Verification items for the finished model (mm, model axes). Face numbers are marked on the shaded views. A direction names the side the tool comes from. Coordinates: 2 decimals unless noted, no trailing zeros. Write each loop counter-clockwise with the first axis right and the second up, starting at its lowest first coordinate (ties: lowest second). Pieces come first, ordered by that corner, then holes. Notation, with made-up numbers: (7, -19) -> (12, -19) arc R32 ccw to (12, 12) -> close; hole circle Ø10 at (49, 45). An arc over 180 degrees is marked (long way). Write item = value, one per line. Start each with the question number.
(1) Mould release check, pull along Y, two halves, no side actions. Record for the marked faces 3, 4, 5 and 6: released by +Y, released by -Y, zero draft, split by the parting line, or undercut.
(2) Section check B-B (x = 11). Record the cut outline in (y, z), plus the area to 3 significant figures.
(3) Section check A-A (y = 21.75). Record the cut outline in (x, z), plus the area to 3 significant figures.
(4) Set-up check for the marked faces 1 and 2: record each of +Z, -Z, +X, -X, +Y, -Y from which the full face is reachable in a straight line by a thin tool's end or side.
(5) Section check C-C (z = -18.75). Record the cut outline in (x, y), plus the area to 3 significant figures.
(6) Gauge pin test, flat end, axial feed: pin 1 Ø2 at (x, z) = (10, -24) entering from -Y. Record the tip position at first contact, or that the pin passes through.
(7) Material ranges on probe 1 along X at (y, z) = (1.95, -7.5); probe 2 along X at (y, z) = (11, -1); probe 3 along X at (y, z) = (23.5, -15.75), recorded low to high. Write a range as [from, to].
(8) Section check D-D (z = -13.75). Record the cut outline in (x, y), plus the area to 3 significant figures.
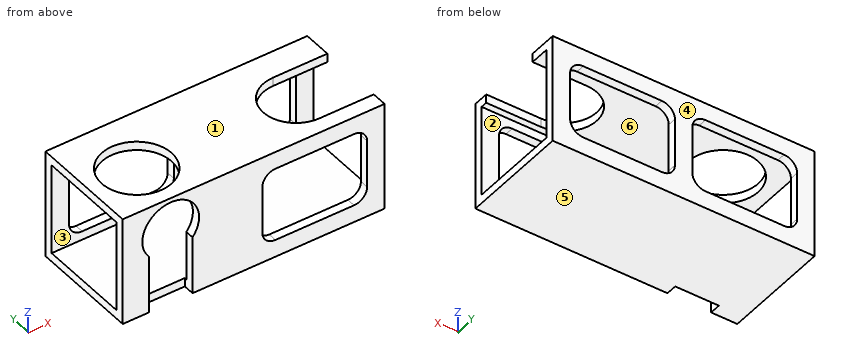
```python
from build123d import *

# Parameters (mm, degrees)
SKETCH_1_W          = 25
SKETCH_1_H          = 25
SKETCH_1_W_2        = 21
SKETCH_1_H_2        = 21
EXTRUDE_1_DEPTH     = 60
CUT_EXTRUDE_1_REACH = 27
SKETCH_2_R          = 8
SKETCH_2_R_2        = 7.5
SKETCH_3_R          = 6.5
CUT_EXTRUDE_2_DEPTH = 4.5
CUT_EXTRUDE_3_DEPTH = 2.5
CUT_EXTRUDE_4_REACH = 27
CUT_EXTRUDE_5_REACH = 27
CUT_EXTRUDE_6_REACH = 27


with BuildPart() as part:
    # Sketch 1 → Extrude 1 (new body)
    with BuildSketch(Plane(origin=(0, 0, 0), x_dir=(0, 0, -1), z_dir=(1, 0, 0))):
        with Locations((12.5, 12.5)):
            Rectangle(SKETCH_1_W, SKETCH_1_H)
        with Locations((12.5, 12.5)):
            Rectangle(SKETCH_1_W_2, SKETCH_1_H_2, mode=Mode.SUBTRACT)
    extrude(amount=EXTRUDE_1_DEPTH)

    # Sketch 2 → Cut-Extrude 1 (cut, up to next)
    with BuildSketch(Plane.XY, mode=Mode.PRIVATE) as cut_extrude_1_sk1:
        with Locations((11, 11)):
            Circle(SKETCH_2_R)
    cut_extrude_1_tool1 = extrude(cut_extrude_1_sk1.sketch, amount=-CUT_EXTRUDE_1_REACH, mode=Mode.PRIVATE) & part.part
    add(cut_extrude_1_tool1.solids().sort_by_distance((11, 11, 0))[0], mode=Mode.SUBTRACT)
    # Sketch 2 → Cut-Extrude 1 (cut, up to next)
    with BuildSketch(Plane.XY, mode=Mode.PRIVATE) as cut_extrude_1_sk2:
        with Locations((47.5, 11)):
            Circle(SKETCH_2_R_2)
    cut_extrude_1_tool2 = extrude(cut_extrude_1_sk2.sketch, amount=-CUT_EXTRUDE_1_REACH, mode=Mode.PRIVATE) & part.part
    add(cut_extrude_1_tool2.solids().sort_by_distance((47.5, 11, 0))[0], mode=Mode.SUBTRACT)

    # Sketch 3 → Cut-Extrude 2 (cut)
    with BuildSketch(Plane.XZ):
        with Locations((11, -7.5)):
            Circle(SKETCH_3_R)
    extrude(amount=-CUT_EXTRUDE_2_DEPTH, mode=Mode.SUBTRACT)

    # Sketch 4 → Cut-Extrude 3 (cut)
    with BuildSketch(Plane(origin=(0, 0, 0), x_dir=(1, 0, 0), z_dir=(0, 1, 0))):
        with BuildLine():
            Line((16, 11.653311931), (16, 25))
            Line((16, 25), (6, 25))
            Line((6, 25), (6, 11.653311931))
            ThreePointArc((6, 11.653311931), (11, 14), (16, 11.653311931))
        make_face()
    extrude(amount=CUT_EXTRUDE_3_DEPTH, mode=Mode.SUBTRACT)

    # Sketch 5 → Cut-Extrude 4 (cut, up to next)
    with BuildSketch(Plane.XY, mode=Mode.PRIVATE) as cut_extrude_4_sk1:
        with BuildLine():
            Line((60, 18.5), (47.5, 18.5))
            ThreePointArc((47.5, 18.5), (52.803300859, 16.303300859), (55, 11))
            ThreePointArc((55, 11), (52.803300859, 5.696699141), (47.5, 3.5))
            Line((47.5, 3.5), (60, 3.5))
            Line((60, 3.5), (60, 18.5))
        make_face()
    cut_extrude_4_tool1 = extrude(cut_extrude_4_sk1.sketch, amount=-CUT_EXTRUDE_4_REACH, mode=Mode.PRIVATE) & part.part
    add(cut_extrude_4_tool1.solids().sort_by_distance((56.483263, 11, 0))[0], mode=Mode.SUBTRACT)

    # Sketch 6 → Cut-Extrude 5 (cut, up to next)
    with BuildSketch(Plane(origin=(0, 25, 0), x_dir=(1, 0, 0), z_dir=(0, 1, 0)), mode=Mode.PRIVATE) as cut_extrude_5_sk1:
        with BuildLine():
            Line((7, 21), (25, 21))
            ThreePointArc((25, 21), (27.121320344, 20.121320344), (28, 18))
            Line((28, 18), (28, 7))
            ThreePointArc((28, 7), (27.121320344, 4.878679656), (25, 4))
            Line((25, 4), (7, 4))
            ThreePointArc((7, 4), (4.878679656, 4.878679656), (4, 7))
            Line((4, 7), (4, 18))
            ThreePointArc((4, 18), (4.878679656, 20.121320344), (7, 21))
        make_face()
    cut_extrude_5_tool1 = extrude(cut_extrude_5_sk1.sketch, amount=-CUT_EXTRUDE_5_REACH, mode=Mode.PRIVATE) & part.part
    add(cut_extrude_5_tool1.solids().sort_by_distance((16, 25, -12.5))[0], mode=Mode.SUBTRACT)
    # Sketch 6 → Cut-Extrude 5 (cut, up to next)
    with BuildSketch(Plane(origin=(0, 25, 0), x_dir=(1, 0, 0), z_dir=(0, 1, 0)), mode=Mode.PRIVATE) as cut_extrude_5_sk2:
        with BuildLine():
            ThreePointArc((53, 21), (55.121320344, 20.121320344), (56, 18))
            Line((56, 18), (56, 7))
            ThreePointArc((56, 7), (55.121320344, 4.878679656), (53, 4))
            Line((53, 4), (35, 4))
            ThreePointArc((35, 4), (32.878679656, 4.878679656), (32, 7))
            Line((32, 7), (32, 18))
            ThreePointArc((32, 18), (32.878679656, 20.121320344), (35, 21))
            Line((35, 21), (53, 21))
        make_face()
    cut_extrude_5_tool2 = extrude(cut_extrude_5_sk2.sketch, amount=-CUT_EXTRUDE_5_REACH, mode=Mode.PRIVATE) & part.part
    add(cut_extrude_5_tool2.solids().sort_by_distance((44, 25, -12.5))[0], mode=Mode.SUBTRACT)

    # Sketch 6_3 → Cut-Extrude 6 (cut, up to next)
    with BuildSketch(Plane(origin=(0, 25, 0), x_dir=(1, 0, 0), z_dir=(0, 1, 0)), mode=Mode.PRIVATE) as cut_extrude_6_sk1:
        with BuildLine():
            ThreePointArc((53, 21), (55.121320344, 20.121320344), (56, 18))
            Line((56, 18), (56, 7))
            ThreePointArc((56, 7), (55.121320344, 4.878679656), (53, 4))
            Line((53, 4), (35, 4))
            ThreePointArc((35, 4), (32.878679656, 4.878679656), (32, 7))
            Line((32, 7), (32, 18))
            ThreePointArc((32, 18), (32.878679656, 20.121320344), (35, 21))
            Line((35, 21), (53, 21))
        make_face()
    cut_extrude_6_tool1 = extrude(cut_extrude_6_sk1.sketch, amount=-CUT_EXTRUDE_6_REACH, mode=Mode.PRIVATE) & part.part
    add(cut_extrude_6_tool1.solids().sort_by_distance((44, 25, -12.5))[0], mode=Mode.SUBTRACT)


solid = part.part
```
Response:
q1.face_3 = undercut
q1.face_4 = released by +Y
q1.face_5 = zero draft
q1.face_6 = undercut
q2.outline = (0, -1) -> (3, -1) -> (3, 0) -> (0, 0) -> close; (2.5, -25) -> (25, -25) -> (25, -21) -> (23, -21) -> (23, -23) -> (2.5, -23) -> close; (19, -2) -> (23, -2) -> (23, -4) -> (25, -4) -> (25, 0) -> (19, 0) -> close
q2.area = 68.0 mm2
q3.outline = (0, -25) -> (60, -25) -> (60, -23) -> (0, -23) -> close; (0, -2) -> (60, -2) -> (60, 0) -> (0, 0) -> close
q3.area = 240 mm2
q4.face_1 = +Z, +X, -X, +Y, -Y
q4.face_2 = +X, -X
q5.outline = (0, 0) -> (6, 0) -> (6, 2) -> (0, 2) -> close; (0, 23) -> (4.1, 23) -> (4.1, 25) -> (0, 25) -> close; (16, 0) -> (32.1, 0) -> (32.1, 2) -> (16, 2) -> close; (27.9, 23) -> (32.1, 23) -> (32.1, 25) -> (27.9, 25) -> close; (55.9, 0) -> (60, 0) -> (60, 2) -> (55.9, 2) -> close; (55.9, 23) -> (60, 23) -> (60, 25) -> (55.9, 25) -> close
q5.area = 77.1 mm2
q6.pin_1 = 2.5
q7.probe_1 = [0, 4.5], [17.5, 32], [56, 60]
q7.probe_2 = [0, 3], [19, 40]
q7.probe_3 = [0, 4], [28, 32], [56, 60]
q8.outline = (0, 0) -> (6, 0) -> (6, 2) -> (0, 2) -> close; (0, 23) -> (4, 23) -> (4, 25) -> (0, 25) -> close; (16, 0) -> (32, 0) -> (32, 2) -> (16, 2) -> close; (28, 23) -> (32, 23) -> (32, 25) -> (28, 25) -> close; (56, 0) -> (60, 0) -> (60, 2) -> (56, 2) -> close; (56, 23) -> (60, 23) -> (60, 25) -> (56, 25) -> close
q8.area = 76.0 mm2
